Autodesk Inventor part; units mm, degrees
ref_plane "YZ Plane" through (0, 0, 0) normal (1, 0, 0) x (0, 1, 0)
ref_plane "XZ Plane" through (0, 0, 0) normal (0, 1, 0) x (-1, 0, 0)
ref_plane "XY Plane" through (0, 0, 0) normal (0, 0, 1) x (1, 0, 0)
ref_plane "Work Plane3" through (0, 1.5, -1.5) normal (0, 0, -1) x (-1, 0, 0)
sketch "Sketch1" plane through (0, 1.5, -1.5) normal (0, 0, -1) x (-1, 0, 0)
  arc A0 (-16, 46) -> (-9, 46) centre (-12.5, 46) ccw
  line L0 (-16, 46) -> (-16, 56)
  arc A1 (-9, 56) -> (-16, 56) centre (-12.5, 56) ccw
  line L1 (-9, 56) -> (-9, 46)
  point P0 (0, -1.5)
extrude "Extrusion1" add sketch "Sketch1" along normal blind 1.5
sketch "Sketch2" plane through (0, 1.5, -1.5) normal (0, 0, 1) x (1, 0, 0)
  line L0 (10.3, 56) -> (10.3, 46)
  arc A0 (10.3, 46) -> (14.7, 46) centre (12.5, 46) ccw
  line L1 (14.7, 46) -> (14.7, 56)
  arc A1 (14.7, 56) -> (10.3, 56) centre (12.5, 56) ccw
  point P0 (0, -1.5)
extrude "Extrusion2" add sketch "Sketch2" along normal blind 2
properties part number "power_button_3DPrint"
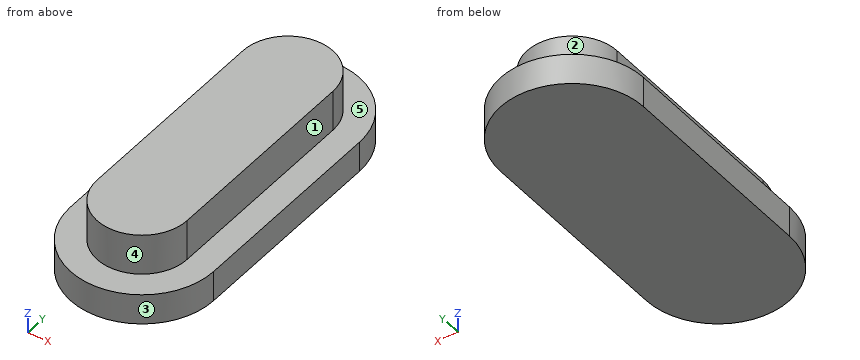
Check sheet for the modelled part. Datum: model origin and axes. Units: mm. Face numbers are marked on the shaded views. A direction names the side the tool comes from. Give positions to 0.01 mm unless a question says otherwise; leave off trailing zeros. Loops run counter-clockwise (first coordinate to the right, second up) from the corner with the lowest first, then second, coordinate; pieces in that order, holes last. Notation, with made-up numbers: M 36.5,-0.5 L 74.5,-0.5 A23 cw 74.5,19.5 Z; hole C 6.5,1.5 d9. An arc over 180 degrees is marked long. Return JSON: item names as keys, results as strings. Group by question number.
1. Cross-section at C-C on z = -0.55. Record the boundary of the cut face in (x, y), plus the area to 3 significant figures.
2. Thickness scan on L1, parallel to Z at x = 15.5, y = 46; L2, parallel to X at y = 48.25, z = -1.05; L3, parallel to X at y = 58, z = -1.75. Record the ranges inside material, lowest first.
3. Cross-section at B-B on x = 12.5. Record the boundary of the cut face in (y, z), plus the area to 3 significant figures.
4. Go/stop test with flat-tipped pins: pin 1 (2 mm diameter, centred on y = 52, z = 0, fed in from +X); pin 2 (0.6 mm diameter, centred on y = 52.5, z = -0.5, fed in from -X); pin 3 (1.5 mm diameter, centred on x = 13.5, z = -1.5, fed in from +Y). Record where each tip stops, or that it passes through.
5. Cross-section at A-A on y = 57.25. Record the boundary of the cut face in (x, z).
6. Cross-section at D-D on z = -1.7. Record the boundary of the cut face in (x, y), plus the area to 3 significant figures.
7. Tool access check on the marked faces 1, 2, 3, 4 and 5. Record the directions out of +Z, -Z, +X, -X, +Y, -Y that give a thin tool (end or side, any length) a straight path to the whole face; none if there is none.
Return value:
{
 "1": {"outline": "M 10.3,47.5 A2.2 ccw 14.7,47.5 L 14.7,57.5 A2.2 ccw 10.3,57.5 Z", "area": "59.2 mm^2"},
 "2": {"L1": "-3 to -1.5", "L2": "10.3 to 14.7", "L3": "9.04 to 15.96"},
 "3": {"outline": "M 44,-3 L 61,-3 L 61,-1.5 L 59.7,-1.5 L 59.7,0.5 L 45.3,0.5 L 45.3,-1.5 L 44,-1.5 Z", "area": "54.3 mm^2"},
 "4": {"pin 1": "x = 14.7", "pin 2": "x = 10.3", "pin 3": "y = 60.99"},
 "5": {"outline": "M 9,-3 L 16,-3 L 16,-1.5 L 14.7,-1.5 L 14.7,0.5 L 10.3,0.5 L 10.3,-1.5 L 9,-1.5 Z"},
 "6": {"outline": "M 9,47.5 A3.5 ccw 16,47.5 L 16,57.5 A3.5 ccw 9,57.5 Z", "area": "108 mm^2"},
 "7": {"face 1": "+Z, +X, +Y, -Y", "face 2": "+Z, +Y", "face 3": "+Z, -Z, -Y", "face 4": "+Z, -Y", "face 5": "+Z"}
}
